from build123d import *

# Parameters (mm, degrees)
F0_R     = 19.05
F1_DEPTH = 31.75
F2_R     = 5.5626
F3_DEPTH = 20.6502
F4_R     = 9.525
F6_DEPTH = 4.7625
F7_R     = 5.5626
F8_DEPTH = 68.2762


with BuildPart() as f1:
    # F0 (on Front) → F1 (new body, symmetric)
    with BuildSketch(Plane.XZ):
        with BuildLine():
            ThreePointArc((0, 31.75), (-22.4506403027, -22.4506403027), (31.75, 0))
            ThreePointArc((31.75, 0), (30.6681449847, 8.217504682), (27.4963065702, 15.875))
            ThreePointArc((27.4963065702, 15.875), (15.875, 27.4963065702), (0, 31.75))
        make_face()
        Circle(F0_R, mode=Mode.SUBTRACT)
        with BuildLine():
            ThreePointArc((0, 31.75), (15.875, 27.4963065702), (27.4963065702, 15.875))
            Line((27.4963065702, 15.875), (50.8, 15.875))
            Line((50.8, 15.875), (50.8, 31.75))
            Line((50.8, 31.75), (0, 31.75))
        make_face()
    extrude(amount=F1_DEPTH, both=True)

    # F2 (on face) → F3 (join)
    with BuildSketch(Plane(origin=(0, 0, 15.875), x_dir=(1, 0, 0), z_dir=(0, 0, -1))):
        with BuildLine():
            Line((90.4493554441, 11.0277214642), (57.0991554441, 30.0777214642))
            ThreePointArc((57.0991554441, 30.0777214642), (44.4246284085, 30.0338352623), (38.1, 19.05))
            Line((38.1, 19.05), (38.1, -19.05))
            ThreePointArc((38.1, -19.05), (44.4246284085, -30.0338352623), (57.0991554441, -30.0777214642))
            Line((57.0991554441, -30.0777214642), (90.4493554441, -11.0277214642))
            ThreePointArc((90.4493554441, -11.0277214642), (96.8502, 0), (90.4493554441, 11.0277214642))
        make_face()
        with Locations((50.8, -19.05)):
            Circle(F2_R, mode=Mode.SUBTRACT)
        with Locations((84.1502, 0)):
            Circle(F2_R, mode=Mode.SUBTRACT)
        with Locations((50.8, 19.05)):
            Circle(F2_R, mode=Mode.SUBTRACT)
    extrude(amount=-F3_DEPTH)

    # F4
    f4_edges = [f1.edges().sort_by_distance(p)[0] for p in [
        (27.496307, 0, 15.875),
    ]]
    fillet(f4_edges, radius=F4_R)

    # F5 (on Front) → F6 (join, symmetric)
    with BuildSketch(Plane.XZ):
        with BuildLine():
            Line((20.0304912791, -24.6341616281), (69.85, 15.875))
            Line((69.85, 15.875), (57.0991554441, 15.875))
            Line((57.0991554441, 15.875), (50.8, 15.875))
            Line((50.8, 15.875), (40.7836134373, 15.875))
            ThreePointArc((40.7836134373, 15.875), (33.5488565837, 12.545475629), (31.3720103364, 4.8846153846))
            ThreePointArc((31.3720103364, 4.8846153846), (29.6377097996, -11.3872146654), (20.0304912791, -24.6341616281))
        make_face()
    extrude(amount=F6_DEPTH, both=True)

    # F7 (on face) → F8 (cut, through all)
    with BuildSketch(Plane.XY.offset(36.5252)):
        with Locations((50.8, 19.05)):
            Circle(F7_R)
        with Locations((50.8, -19.05)):
            Circle(F7_R)
    extrude(amount=-F8_DEPTH, mode=Mode.SUBTRACT)


solid = f1.part
Geometry check sheet. Reference: the model listing, model coordinates, mm. A direction names the side the tool comes from. Give positions to 0.01 mm unless a question says otherwise; leave off trailing zeros. Loops run counter-clockwise (first coordinate to the right, second up) from the corner with the lowest first, then second, coordinate; pieces in that order, holes last. Notation, with made-up numbers: (83, -1) -> (133, -1) arc R11 cw to (133, 3) -> close; hole circle Ø6 at (-1, 25). An arc over 180 degrees is marked (long way). Answer in a Markdown table with one row per item. Add a question column.
1) Cross-section at C-C on z = 0. Record the boundary of the cut face in (x, y), and give its area (3 significant figures).
2) Set-up check for faces 1 (the face through (62, -8, 15.875)), 2 (the face through (33.62, 18.45, 12.63)), 3 (the face through (33.62, -18.07, 12.63)): record each of +Z, -Z, +X, -X, +Y, -Y from which the full face is reachable in a straight line by a thin tool's end or side.
3) Gauge pin test, flat ends, axial feed: P1, Ø2, axis at x = 60, z = 28.5, coming from the +Y side; P2, Ø5, axis at x = 27, y = -21, coming from the +Z side; P3, Ø1, axis at x = 57, z = 21.5, coming from the +Y side; P4, Ø13, axis at x = 84.15, y = 0, coming from the +Z side. Record the tip position at first contact, or that the pin passes through.
4) Cross-section at B-B on x = -12. Record the boundary of the cut face in (y, z), and give its area (3 significant figures).
5) Material ranges on probe 1 along Y at (x, z) = (50.8, 24.5); probe 2 along Z at (x, y) = (0, 16.5); probe 3 along Y at (x, z) = (50, 31), recorded low to high. Write a range as from..to.
6) Cross-section at D-D on z = 24.5. Record the boundary of the cut face in (x, y).
7) Cross-section at A-A on y = 0. State how many separate pieces and enclosed holes the cut face has, and give its area (3 significant figures).
8) Draft check along Y on faces 4 (the face through (56.106, 17.379, 26.056)), 5 (the face through (61, 0, 36.525)), 6 (the face through (78.593, -0.245, 26.056)), 7 (the face through (43, -4.762, 2)). Enter one of: pulls with the +Y half, pulls with the -Y half, needs draft (parallel to the pull), parting line crosses it, or undercut.
Outcome:
| question | item | result |
|---|---|---|
| 1 | outline | (-31.75, -31.75) -> (-19.05, -31.75) -> (-19.05, 31.75) -> (-31.75, 31.75) -> close; (19.05, -31.75) -> (31.75, -31.75) -> (31.75, -4.76) -> (50.33, -4.76) -> (50.33, 4.76) -> (31.75, 4.76) -> (31.75, 31.75) -> (19.05, 31.75) -> close |
| 1 | area | 1,790 mm^2 |
| 2 | face 1 | -Z, +X |
| 2 | face 2 | +X, +Y |
| 2 | face 3 | +X, -Y |
| 3 | P1 | stops at y = 28.99 |
| 3 | P2 | stops at z = 31.75 |
| 3 | P3 | stops at y = 30.4 |
| 3 | P4 | stops at z = 36.53 |
| 4 | outline | (-31.75, -29.39) -> (31.75, -29.39) -> (31.75, -14.8) -> (-31.75, -14.8) -> close; (-31.75, 14.8) -> (31.75, 14.8) -> (31.75, 29.39) -> (-31.75, 29.39) -> close |
| 4 | area | 1,850 mm^2 |
| 5 | probe 1 | y = -31.75..-24.61, -13.49..13.49, 24.61..31.75 |
| 5 | probe 2 | z = -31.75..-19.05, 19.05..31.75 |
| 5 | probe 3 | y = -31.75..-24.55, -13.55..13.55, 24.55..31.75 |
| 6 | outline | (-20.19, -31.75) -> (50.8, -31.75) arc R12.7 ccw to (57.1, -30.08) -> (90.45, -11.03) arc R12.7 ccw to (90.45, 11.03) -> (57.1, 30.08) arc R12.7 ccw to (50.8, 31.75) -> (-20.19, 31.75) -> close; hole circle Ø11.13 at (50.8, -19.05); hole circle Ø11.13 at (50.8, 19.05); hole circle Ø11.13 at (84.15, 0) |
| 7 | separate pieces | 2 |
| 7 | enclosed holes | 1 |
| 7 | area | 3,950 mm^2 |
| 8 | face 4 | undercut |
| 8 | face 5 | needs draft |
| 8 | face 6 | undercut |
| 8 | face 7 | pulls with the -Y half |
